from build123d import *

# Parameters (mm, degrees)
FILLET2_R          = 1
CHAMFER1_SIZE      = 0.3
SKETCH2_R          = 1.5
CUT_EXTRUDE1_DEPTH = 10
SKETCH3_R          = 2.75
CUT_EXTRUDE2_DEPTH = 10


with BuildPart() as part:
    # Sketch1 → Revolve1 (revolve)
    with BuildSketch(Plane.XY, mode=Mode.PRIVATE) as revolve1_sk:
        with BuildLine():
            Line((-10, 7), (-10, 11))
            Line((-10, 11), (-6, 11))
            Line((-6, 11), (-6, 18.5))
            Line((-6, 18.5), (-4.655646626, 18.5))
            ThreePointArc((-4.655646626, 18.5), (-4.107342929, 18.336279293), (-3.73857657, 17.898726111))
            Line((-3.73857657, 17.898726111), (0.170700563, 8.907388706))
            ThreePointArc((0.170700563, 8.907388706), (0.790480214, 6.956422558), (1, 4.920127592))
            Line((1, 4.920127592), (1, 0))
            Line((1, 0), (-2, 0))
            Line((-2, 0), (-2, 7))
            Line((-2, 7), (-10, 7))
        make_face()
    revolve(revolve1_sk.sketch.rotate(Axis((0, 0, 0), (1, 0, 0)), 90), axis=Axis((0, 0, 0), (1, 0, 0)))

    # Fillet2
    fillet2_edges = [part.edges().sort_by_distance(p)[0] for p in [
        (-6, 0, -11),
        (-2, 0, -7),
    ]]
    fillet(fillet2_edges, radius=FILLET2_R)

    # Chamfer1
    chamfer1_edges = [part.edges().sort_by_distance(p)[0] for p in [
        (-6, 0, -18.5),
        (-10, 0, -11),
    ]]
    chamfer(chamfer1_edges, length=CHAMFER1_SIZE)

    # Sketch2 → Cut-Extrude1 (cut)
    with BuildSketch(Plane.ZY.offset(6)):
        with Locations((0, 14.5)):
            Circle(SKETCH2_R)
        with Locations((14.5, 0)):
            Circle(SKETCH2_R)
        with Locations((0, -14.5)):
            Circle(SKETCH2_R)
        with Locations((-14.5, 0)):
            Circle(SKETCH2_R)
    extrude(amount=-CUT_EXTRUDE1_DEPTH, mode=Mode.SUBTRACT)

    # Sketch3 → Cut-Extrude2 (cut)
    with BuildSketch(Plane.ZY.offset(4)):
        with Locations((0, 14.5)):
            Circle(SKETCH3_R)
        with Locations((14.5, 0)):
            Circle(SKETCH3_R)
        with Locations((0, -14.5)):
            Circle(SKETCH3_R)
        with Locations((-14.5, 0)):
            Circle(SKETCH3_R)
    extrude(amount=-CUT_EXTRUDE2_DEPTH, mode=Mode.SUBTRACT)


solid = part.part
Input: part model. Units: mm. Frame: model coordinates. A direction names the side the tool comes from. Give positions to 0.01 mm unless a question says otherwise; leave off trailing zeros. Use one line per item in the form item = value.
1. Mould query, pull axis Y, two halves, no side actions, for faces 4 (the face through (-6, -12.4, 0.3)), 5 (the face through (-4, 13, 1)), 6 (the face through (-8.33, 10.74, -2.38)), 7 (the face through (-4, -16, 1)). Classes: released by +Y, released by -Y, zero draft, split by the parting line, or undercut.
Outcome:
face_4 = zero draft
face_5 = undercut
face_6 = split by the parting line
face_7 = undercut
2. Cut plane A-A on z = 0. State how many separate pieces and enclosed holes the cut face has, and give its area (3 significant figures).
Outcome:
separate_pieces = 3
enclosed_holes = 0
area = 146 mm²
3. Reachability of faces 1 (the face through (-2, 0, 0)), 2 (the face through (-2.879, -11.773, -0.358)), 3 (the face through (-5, 0, 13)) from +Z, -Z, +X, -X, +Y, -Y: full face, straight path, thin tool, end or side. Return the list, or none.
Outcome:
face_1 = -X
face_2 = +X
face_3 = +X, -X
4. First-contact query: P1, Ø1.5, axis at x = -6, y = 4.5, coming from the +Z side; P2, Ø3, axis at x = -3, z = -4.5, coming from the -Y side; P3, Ø6, axis at y = -13.5, z = 6, coming from the +X side; P4, Ø2.5, axis at y = 14.5, z = 0, coming from the -X side. Flat tips, straight axial feed; report the tip coordinate or a pass-through.
Outcome:
P1 = 18.1
P2 = -18.05
P3 = -1.08
P4 = through
5. Ray query, L1, parallel to Y at x = -5.25, z = 0; L2, parallel to Y at x = -3.4, z = 0; L3, parallel to Y at x = -2.1, z = 0. Return the intervals inside material, ascending.
Outcome:
L1 = -18.5 to -16, -13 to -7, 7 to 13, 16 to 18.5
L2 = -11.75 to -7, 7 to 11.75
L3 = -11.75 to -6.44, 6.44 to 11.75
